Can you work these out from the drawing? Everything is in mm from the part's minimum corner. A direction names the side the tool comes from. Give positions to 0.01 mm unless a question says otherwise; leave off trailing zeros. Order: outer loops, then holes, each group sorted by start corner. A loop starts at its lowest first (then second) coordinate and runs counter-clockwise, first axis right, second up. Notation, with made-up numbers: M 1,-40 L 28,-40 A21 ccw 28,-17 Z; hole C -33,-8 d6. An arc over 180 degrees is marked long. Answer as a JSON object with one key per item and string values.
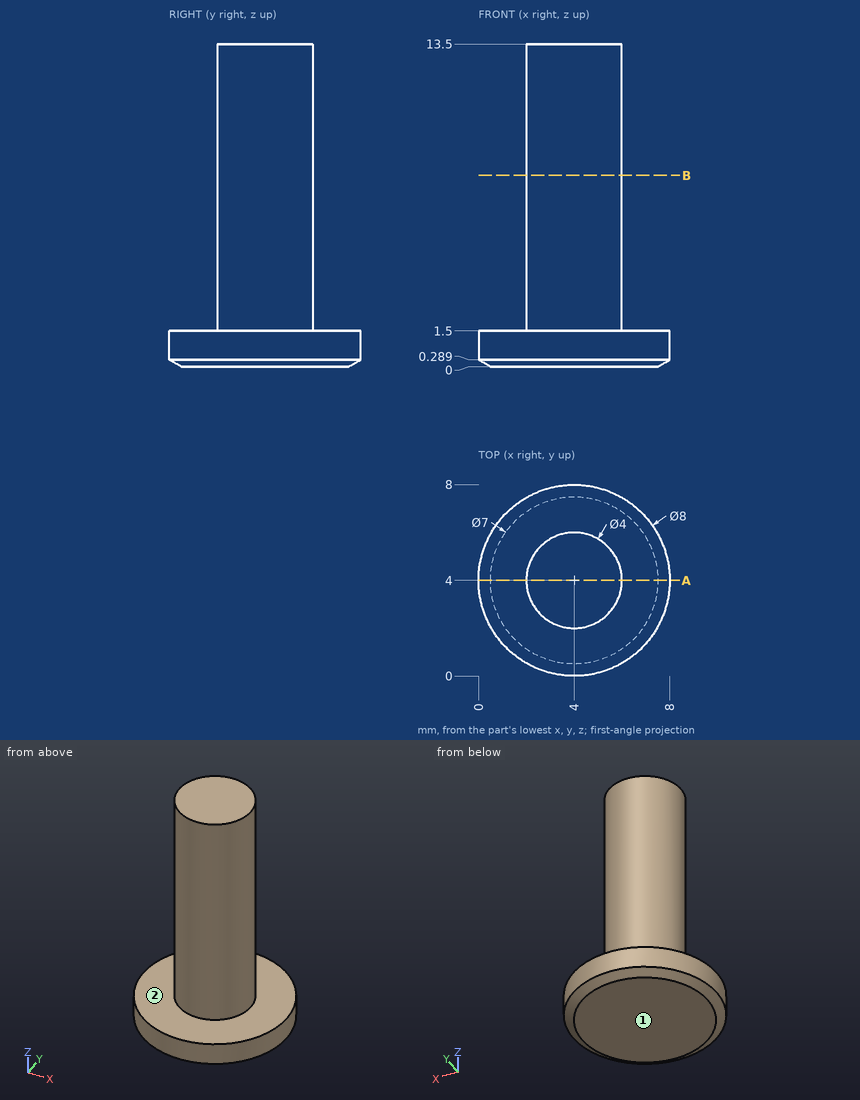
1) I want a section at A-A on y = 4. Write out the boundary of the cut face in (x, z).
Results found:
{"outline": "M 0,0.29 L 0.5,0 L 7.5,0 L 8,0.29 L 8,1.5 L 6,1.5 L 6,13.5 L 2,13.5 L 2,1.5 L 0,1.5 Z"}
2) I need wall thicknesses on L1, parallel to Z at x = 5.25, y = 1.75; L2, parallel to Y at x = 3.25, z = 5 (1 decimal); L3, parallel to Y at x = 2.25, z = 11. Which ranges of each line are inside material? Lowest first, please.
Results found:
{"L1": "z = 0 to 1.5", "L2": "y = 2.1 to 5.9", "L3": "y = 3.03 to 4.97"}
3) I want a section at B-B on z = 8. Write out the boundary of the cut face in (x, y), and give its area (3 significant figures).
Results found:
{"outline": "C 4,4 d4", "area": "12.6 mm²"}
4) For the marked faces 1 and 2, which set-ups out of +Z, -Z, +X, -X, +Y, -Y let a thin tool reach every point of the face, with its end or its side?
Results found:
{"face 1": "-Z, +X, -X, +Y, -Y", "face 2": "+Z"}
5) I'm going to push flat-ended pins straight in: pin 1 Ø1.5 at (x, z) = (6, 10.5) entering from -Y; pin 2 Ø1 at (y, z) = (6, 6.5) entering from -X; pin 3 Ø1 at (x, z) = (2, 8.5) entering from -Y. Where does each tip first touch, or does it pass through?
Results found:
{"pin 1": "stops at y = 2.44", "pin 2": "stops at x = 2.68", "pin 3": "stops at y = 2.68"}
